Model file for the job. Use its own axes, mm. A direction names the side the tool comes from. Coordinates: 2 decimals unless noted, no trailing zeros. Order: outer loops, then holes, each group sorted by start corner. A loop starts at its lowest first (then second) coordinate and runs counter-clockwise, first axis right, second up.
from build123d import *

# Parameters (mm, degrees)
BOSS_EXTRUDE1_DEPTH = 3
SKETCH2_W           = 11
SKETCH2_H           = 8
BOSS_EXTRUDE2_DEPTH = 12
SKETCH4_R           = 1.5
BOSS_EXTRUDE4_DEPTH = 5
BOSS_EXTRUDE5_DEPTH = 5
SKETCH3_R           = 1.5
BOSS_EXTRUDE3_DEPTH = 2
BOSS_EXTRUDE6_DEPTH = 2


with BuildPart() as part:
    # Sketch1 → Boss-Extrude1 (new body)
    with BuildSketch(Plane(origin=(0, 0, 0), x_dir=(1, 0, 0), z_dir=(0, 1, 0))):
        with BuildLine():
            Line((-1.1, 1.487447478), (-1.1, -1.487447478))
            ThreePointArc((-1.1, -1.487447478), (1.85, 0), (-1.1, 1.487447478))
        make_face()
    extrude(amount=BOSS_EXTRUDE1_DEPTH)

    # Sketch2 → Boss-Extrude2 (add)
    with BuildSketch(Plane(origin=(0, 3, 0), x_dir=(1, 0, 0), z_dir=(0, 1, 0))):
        with Locations((-3.65, 0)):
            Rectangle(SKETCH2_W, SKETCH2_H)
    extrude(amount=BOSS_EXTRUDE2_DEPTH)

    # Sketch4 → Boss-Extrude4 (add)
    with BuildSketch(Plane(origin=(0, 15, 0), x_dir=(1, 0, 0), z_dir=(0, 1, 0))):
        with Locations(Location((0, 0, 0), (0, 0, 270))):
            Circle(SKETCH4_R)
    extrude(amount=BOSS_EXTRUDE4_DEPTH)

    # Sketch5 → Boss-Extrude5 (add, symmetric)
    with BuildSketch(Plane.XY):
        with BuildLine():
            Line((-9.15, 13.177050983), (-9.15, 9.822949017))
            ThreePointArc((-9.15, 9.822949017), (-5.4, 11.5), (-9.15, 13.177050983))
        make_face()
    extrude(amount=BOSS_EXTRUDE5_DEPTH, both=True)

    # Sketch3 → Boss-Extrude3 (add)
    with BuildSketch(Plane.XY.offset(5)):
        with Locations(Location((-7.65, 11.5, 0), (0, 0, 180))):
            Circle(SKETCH3_R)
    extrude(amount=BOSS_EXTRUDE3_DEPTH)

    # Sketch6 → Boss-Extrude6 (add)
    with BuildSketch(Plane(origin=(0, 0, -5), x_dir=(-1, 0, 0), z_dir=(0, 0, -1))):
        with BuildLine():
            Line((8.75, 10.075219315), (8.75, 12.924780685))
            ThreePointArc((8.75, 12.924780685), (5.85, 11.5), (8.75, 10.075219315))
        make_face()
    extrude(amount=BOSS_EXTRUDE6_DEPTH)


solid = part.part
Q1. Cut at B-B, the plane y = 2.5. List the corners of the cut face in (x, z), plus the area to 3 significant figures.
Established:
outline: (-1.1, -1.49) arc R1.85 ccw (long way) to (-1.1, 1.49) - close
area: 9.19 mm2
Q2. Drop flat-ended pins along their axis: P1, Ø2.5, axis at x = -4.5, z = 0.5, coming from the +Y side; P2, Ø2, axis at y = 17.5, z = 0.5, coming from the -X side; P3, Ø1, axis at x = -3.5, y = 11, coming from the -Z side; P4, Ø2, axis at y = 12, z = -5.5, coming from the -X side. Give the stop position or say it passes through.
Established:
P1: stops at y = 15
P2: stops at x = -1.5
P3: stops at z = -4
P4: stops at x = -9.15
Q3. Which spindle directions (+Z, -Z, +X, -X, +Y, -Y) get a long thin tool onto all of the face, cutting with end or side? Do faces 1 (the face through (-9, 11, -5)), 2 (the face through (-5.4, 11.43, 4.51)), 3 (the face through (1.85, 1.48, 0.06)). Say none if no direction does.
Established:
face 1: -Z
face 2: +Z
face 3: -Y
Q4. Cut at D-D, the plane x = 0. List the corners of the cut face in (y, z).
Established:
outline: (0, -1.85) - (3, -1.85) - (3, -4) - (15, -4) - (15, -1.5) - (20, -1.5) - (20, 1.5) - (15, 1.5) - (15, 4) - (3, 4) - (3, 1.85) - (0, 1.85) - close
Q5. Cut at A-A, the plane x = -7.65. List the corners of the cut face in (y, z), plus the area to 3 significant figures.
Established:
outline: (3, -4) - (9.25, -4) - (9.25, -5) - (9.7, -5) - (9.7, -7) - (13.3, -7) - (13.3, -5) - (13.75, -5) - (13.75, -4) - (15, -4) - (15, 4) - (13.75, 4) - (13.75, 5) - (13, 5) - (13, 7) - (10, 7) - (10, 5) - (9.25, 5) - (9.25, 4) - (3, 4) - close
area: 118 mm2
Q6. Probe line 1 (Z direction, x = 0, y = 11.75); line 2 (Y direction, x = -3.5, z = -3.25); line 3 (Z direction, x = 0.25, y = 1.25). List the from-to ranges inside material, lowest first.
Established:
line 1: z = -4 to 4
line 2: y = 3 to 15
line 3: z = -1.83 to 1.83
Q7. Cut at C-C, the plane z = -0.5. List the corners of the cut face in (x, y).
Established:
outline: (-9.15, 3) - (-1.1, 3) - (-1.1, 0) - (1.78, 0) - (1.78, 3) - (1.85, 3) - (1.85, 15) - (1.41, 15) - (1.41, 20) - (-1.41, 20) - (-1.41, 15) - (-9.15, 15) - close
